Design review of the part built by this model. Coordinates are the model's own, in mm. Face numbers are marked on the shaded views. A direction names the side the tool comes from. Give positions to 0.01 mm unless a question says otherwise; leave off trailing zeros. Order: outer loops, then holes, each group sorted by start corner. A loop starts at its lowest first (then second) coordinate and runs counter-clockwise, first axis right, second up. Notation, with made-up numbers: (82, 60) - (130, 60) arc R21 cw to (130, 78) - close; hole circle Ø5 at (59.5, 34). An arc over 180 degrees is marked (long way). Write each question's results on one line, items separated by ' | '. Start each with the question number.
```python
from build123d import *

# Parameters (mm, degrees)
F1_DEPTH = 38.1
F3_DEPTH = 12.701


with BuildPart() as f1:
    # F0 (on Right) → F1 (new body)
    with BuildSketch(Plane.YZ):
        Polygon((0, 0), (0, 31.75), (-12.7, 31.75), (-12.7, 12.7), (-25.4, 12.7), (-25.4, 0), align=None)
    extrude(amount=F1_DEPTH)

    # F2 (on face) → F3 (cut, through all)
    with BuildSketch(Plane.XZ.offset(12.7)):
        Polygon((25.318417, 31.75), (12.966445, 31.75), (12.618417, 25.409544), (25.318417, 25.409544), align=None)
    extrude(amount=-F3_DEPTH, mode=Mode.SUBTRACT)


solid = f1.part
```
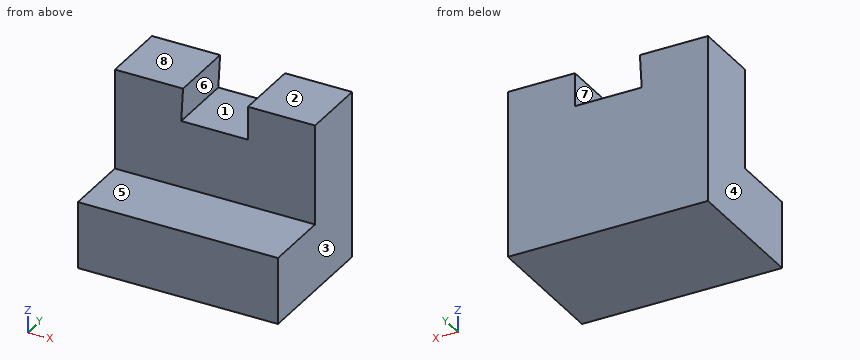
Q1. Add section B-B (x = 28). Give the boundary of the cut face in (y, z).
Q2. Add section C-C (z = 17). Give the boundary of the cut face in (x, y).
Q3. Machinability: for the marked faces 5, 6, 7 and 8, which of the approach directions +Z, -Z, +X, -X, +Y, -Y give a long, thin tool a straight path to every point of the face, cutting with its end or side? Answer none if there is none.
Q4. Insertion check: pin 1 Ø4 at (x, y) = (16, -9.5) entering from +Z; pin 2 Ø6 at (x, y) = (8, -21) entering from +Z; pin 3 Ø2 at (x, z) = (7.5, 14.5) entering from -Y. Each pin has a flat end and moves straight along its axis. Give the tip position at first contact, or say it passes through.
Q5. Add section A-A (y = -11.5). Give the boundary of the cut face in (x, z).
Q6. For line 1 (Z direction, x = 18, y = -13.75); line 2 (Y direction, x = 10, z = 28); line 3 (Z direction, x = 13, y = -4), list the stretches that pass through material, from the lowest coordinate up. Write a range as [from, to].
Q7. Draft analysis for pull direction X (two halves, no side actions). For the marked faces 1, 2, 3 and 4, state which applies: pulls with the +X half, pulls with the -X half, needs draft (parallel to the pull), parting line crosses it, or undercut.
Q8. Add section D-D (x = 23). Give the boundary of the cut face in (y, z), plus the area to 3 significant figures.
Verdict:
1) outline: (-25.4, 0) - (0, 0) - (0, 31.75) - (-12.7, 31.75) - (-12.7, 12.7) - (-25.4, 12.7) - close
2) outline: (0, -12.7) - (38.1, -12.7) - (38.1, 0) - (0, 0) - close
3) face 5: +Z, +X, -X, -Y | face 6: +Y, -Y | face 7: +Z, +Y, -Y | face 8: +Z, +X, -X, +Y, -Y
4) pin 1: stops at z = 25.41 | pin 2: stops at z = 12.7 | pin 3: stops at y = -12.7
5) outline: (0, 0) - (38.1, 0) - (38.1, 31.75) - (25.32, 31.75) - (25.32, 25.41) - (12.62, 25.41) - (12.97, 31.75) - (0, 31.75) - close
6) line 1: z = [0, 12.7] | line 2: y = [-12.7, 0] | line 3: z = [0, 25.41]
7) face 1: undercut | face 2: needs draft | face 3: pulls with the +X half | face 4: pulls with the -X half
8) outline: (-25.4, 0) - (0, 0) - (0, 25.41) - (-12.7, 25.41) - (-12.7, 12.7) - (-25.4, 12.7) - close | area: 484 mm2
